The model under review builds one solid part; all positions refer to its coordinate system, in mm. A direction names the side the tool comes from. Coordinates: 2 decimals unless noted, no trailing zeros. Order: outer loops, then holes, each group sorted by start corner. A loop starts at its lowest first (then second) coordinate and runs counter-clockwise, first axis right, second up. Notation, with made-up numbers: (81, 13.25) - (98, 13.25) arc R26 ccw to (98, 45.25) - close; hole circle Ø10 at (-31, 66.5). An arc over 180 degrees is marked (long way). Answer in a Markdown table with one row per item.
Autodesk Inventor part; units mm, degrees
ref_plane "Work Plane1" through (0, -862.1118, 0) normal (0, 0, 1) x (-1, 0, 0)
ref_plane "YZ Plane" through (0, 0, 0) normal (1, 0, 0) x (0, 1, 0)
ref_plane "XZ Plane" through (0, 0, 0) normal (0, 1, 0) x (-1, 0, 0)
ref_plane "Work Plane1" through (0, -862.1118, 0) normal (0, 0, 1) x (-1, 0, 0)
sketch "Sketch1" plane through (0, -862.1118, 0) normal (0, 0, 1) x (-1, 0, 0)
  circle A0 centre (-188, -18) radius 4
  line L0 (-220, -478) -> (-220, 22)
  line L1 (-220, -478) -> (-208, -478)
  line L2 (-208, 22) -> (-208, -478)
  line L3 (-220, 22) -> (-208, 22)
  line L4 (-208, -27.0151) -> (-198, -27.0151)
  line L5 (-198, -107.0151) -> (-208, -107.0151)
  line L6 (-208, -107.0151) -> (-208, -27.0151)
  line L7 (-155, -45.5151) -> (-198, -45.5151)
  line L8 (-198, -88.5151) -> (-155, -88.5151)
  line L9 (-155, -88.5151) -> (-155, -45.5151)
  circle A1 centre (-176.15, -66.6651) radius 11.5
  circle A2 centre (-161, -51.5151) radius 2
  circle A3 centre (-192, -51.5151) radius 2
  circle A4 centre (-192, -82.5151) radius 2
  circle A5 centre (-161, -82.5151) radius 2
  line L10 (-192, -82.5151) -> (-192, -51.5151) construction
  line L11 (-192, -82.5151) -> (-161, -82.5151) construction
  line L12 (-198, -27.0151) -> (-198, -45.5151)
  line L13 (-198, -88.5151) -> (-198, -107.0151)
  point P0 (0, -862.1118)
  dimension "d0" = 10
  dimension "d1" = 80
  dimension "d3" = 43
  dimension "d4" = 18.5
  dimension "d5" = 18.5
  dimension "d6" = 23
  dimension "d7" = 4
  dimension "d8" = 4
  dimension "d9" = 4
  dimension "d10" = 4
  dimension "d11" = 31
  dimension "d12" = 31
  dimension "d13" = 31
  dimension "d14" = 31
  dimension "d15" = 6
  dimension "d18" = 6
  dimension "d19" = 6
  dimension "d20" = 6
  dimension "d21" = 90
  dimension "d25" = 21.15
  dimension "d26" = 21.15
  dimension "d27" = 90
  dimension "d28" = 90
  dimension "d29" = 18.5
extrude "Tykkelse" add sketch "Sketch1" along normal blind 20 contours L2 L4 L12 L7 L9 L8 L13 L5
sketch "Sketch2" plane through (198, -835.0967, 0) normal (-1, 0, 0) x (0, 0, 1)
  line L0 (0, 0) -> (20, 0)
  line L1 (20, 18.5) -> (20, 0)
  line L2 (0, 80) -> (0, 61.5)
  line L3 (0, 61.5) -> (20, 61.5)
  line L4 (20, 80) -> (20, 61.5)
  line L5 (0, 80) -> (20, 80)
  circle A0 centre (10, 70) radius 3.5
  circle A1 centre (10, 10) radius 3.5
  point P0 (0, 835.0967)
  dimension "d32" = 7
  dimension "d33" = 7
  dimension "d34" = 10
  dimension "d35" = 10
  dimension "d36" = 10
  dimension "d37" = 10
extrude "Extrusion2" cut sketch "Sketch2" against normal up to surface (10 mm away) contours A0 | A1
fillet "Fillet1" radius 0.5 8 edges at (198, -816.5967, 10) (198, -773.5967, 10) (155, -773.5967, 10) (155, -816.5967, 10) (198, -835.0967, 10) (208, -835.0967, 10) (198, -755.0967, 10) (208, -755.0967, 10)
equation "\"d4\" = d5"
equation "\"d8\" = d7"
equation "\"d9\" = d7"
equation "\"d10\" = d7"
equation "\"d13\" = d11"
equation "\"d14\" = d12"
equation "\"d15\" = d20"
equation "\"d18\" = d15"
equation "\"d19\" = d18"
properties part number "Stepper Holder X&Y" material "Aluminum 6061"
Item 1: Tool access review of faces 4 (the face through (177, -773.597, 10)), 5 (the face through (188, -796, 20)), 6 (the face through (176, -816.597, 10)): name each direction out of +Z, -Z, +X, -X, +Y, -Y from which nothing blocks a thin tool from reaching the whole face with its end or side.
Check values:
| item | result |
|---|---|
| face 4 | +Z, -Z, -X, +Y |
| face 5 | +Z, +X, -X, +Y, -Y |
| face 6 | +Z, -Z, -X, -Y |
Item 2: We need section B-B, the plane z = 7.75. State how many separate pieces and enclosed holes the cut face has, then the cut area to 3 significant figures.
Check values:
| item | result |
|---|---|
| separate pieces | 3 |
| enclosed holes | 5 |
| area | 2,080 mm^2 |
Item 3: We need section C-C, the plane x = 192. Write out the cut boundary in (y, z), then the cut area to 3 significant figures.
Check values:
| item | result |
|---|---|
| outline | (-816.6, 0) - (-812.6, 0) - (-812.6, 20) - (-816.6, 20) - close; (-808.6, 0) - (-781.6, 0) - (-781.6, 20) - (-808.6, 20) - close; (-777.6, 0) - (-773.6, 0) - (-773.6, 20) - (-777.6, 20) - close |
| area | 700 mm^2 |
Item 4: We need section A-A, the plane x = 176.15. Write out the cut boundary in (y, z), then the cut area to 3 significant figures.
Check values:
| item | result |
|---|---|
| outline | (-816.6, 0) - (-806.95, 0) - (-806.95, 20) - (-816.6, 20) - close; (-783.95, 0) - (-773.6, 0) - (-773.6, 20) - (-783.95, 20) - close |
| area | 400 mm^2 |
Item 5: Clearance check with flat-ended pins moving along their axes: pin 1 Ø8 at (y, z) = (-765.1, 10) entering from -X; pin 2 Ø2 at (x, y) = (187, -784.5) entering from -Z; pin 3 Ø3 at (x, z) = (172, 8.5) entering from -Y; pin 4 Ø3 at (x, y) = (192, -779.6) entering from -Z. State where each tip first meets the part, or that it passes through.
Check values:
| item | result |
|---|---|
| pin 1 | x = 198 |
| pin 2 | z = 0 |
| pin 3 | y = -816.6 |
| pin 4 | through |
Item 6: To check wall thickness, follow line 1 (Y direction, x = 161, z = 12.5); line 2 (Y direction, x = 201.5, z = 10); line 3 (Y direction, x = 176.15, z = 15.5). State the ranges of each line that lie inside material, in increasing order. Write a range as from..to.
Check values:
| item | result |
|---|---|
| line 1 | -816.6..-812.6, -808.6..-781.6, -777.6..-773.6 |
| line 2 | -835.1..-828.6, -821.6..-768.6, -761.6..-755.1 |
| line 3 | -816.6..-806.95, -783.95..-773.6 |
Item 7: Mouldability with a two-part tool opening along Y and no side actions: class faces 1 (the face through (203, -835.097, 10)), 2 (the face through (161.26, -808.614, 9.86)), 3 (the face through (198, -827.9, 7.6)) as +Y half, -Y half, draft (parallel to the pull), parting line (faces both ways), or undercut.
Check values:
| item | result |
|---|---|
| face 1 | -Y half |
| face 2 | undercut |
| face 3 | draft |
Item 8: We need section D-D, the plane y = -799.5. Write out the cut boundary in (x, z).
Check values:
| item | result |
|---|---|
| outline | (155, 0) - (165.39, 0) - (165.39, 20) - (155, 20) - close; (186.91, 0) - (208, 0) - (208, 20) - (186.91, 20) - close |
